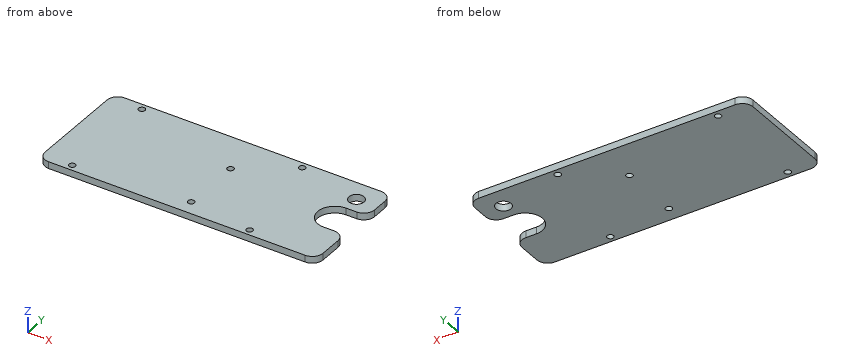
from build123d import *

# Parameters (mm, degrees)
F0_R     = 3.5
F1_DEPTH = 3.175
F3_R     = 5
F2_R     = 1.5
F4_DEPTH = 25


with BuildPart() as f1:
    # F0 (on Top) → F1 (new body)
    with BuildSketch(Plane.XY):
        with BuildLine():
            Line((65, 27), (-65, 27))
            Line((-65, 27), (-65, -27))
            Line((-65, -27), (65, -27))
            Line((65, -27), (65, -6.4))
            Line((65, -6.4), (55, -6.4))
            ThreePointArc((55, -6.4), (47, 1.6), (55, 9.6))
            Line((55, 9.6), (65, 9.6))
            Line((65, 9.6), (65, 27))
        make_face()
        with Locations((55, 17)):
            Circle(F0_R, mode=Mode.SUBTRACT)
    extrude(amount=F1_DEPTH)

    # F3
    f3_edges = [f1.edges().sort_by_distance(p)[0] for p in [
        (-65, -27, 1.5875),
        (-65, 27, 1.5875),
        (65, -27, 1.5875),
        (65, -6.4, 1.5875),
        (65, 9.6, 1.5875),
        (65, 27, 1.5875),
    ]]
    fillet(f3_edges, radius=F3_R)

    # F2 (on face) → F4 (cut)
    with BuildSketch(Plane.XY.offset(3.175)):
        with Locations((25, 24)):
            Circle(F2_R)
        with Locations((2, 8)):
            Circle(F2_R)
        with Locations((32, -24)):
            Circle(F2_R)
        with Locations((2, -20)):
            Circle(F2_R)
        with Locations((-50, 24)):
            Circle(F2_R)
        with Locations((-51, -24)):
            Circle(F2_R)
    extrude(amount=-F4_DEPTH, mode=Mode.SUBTRACT)


solid = f1.part
Could you check a few things on this model? Use its own coordinates, in mm. Round coordinates to 2 decimals unless told otherwise and drop trailing zeros. Loops run counter-clockwise (first coordinate to the right, second up) from the corner with the lowest first, then second, coordinate; pieces in that order, holes last. Notation, with made-up numbers: (-12, 33) -> (35, 33) arc R20 cw to (35, 47) -> close; hole circle Ø9 at (-24.75, 43). An arc over 180 degrees is marked (long way). Use CSV: the item, a comma, the result in double quotes.
(1) Suppose I cut it at B-B on x = 2. Write out the boundary of the cut face in (y, z) (3 decimals), plus the area to 3 significant figures.
Return value:
outline,"(-27, 0) -> (-21.5, 0) -> (-21.5, 3.175) -> (-27, 3.175) -> close; (-18.5, 0) -> (6.5, 0) -> (6.5, 3.175) -> (-18.5, 3.175) -> close; (9.5, 0) -> (27, 0) -> (27, 3.175) -> (9.5, 3.175) -> close"
area,"152 mm²"
(2) If I drill on probe 1 along Y at (x, z) = (55, 1.8); probe 2 along Y at (x, z) = (2, 2.25); probe 3 along Y at (x, z) = (59.5, 2.9), over which ranges is the centre line in solid material (lowest first)? Write a range as [from, to].
Return value:
probe 1,"y = [-27, -6.4], [9.6, 13.5], [20.5, 27]"
probe 2,"y = [-27, -21.5], [-18.5, 6.5], [9.5, 27]"
probe 3,"y = [-27, -6.4], [9.6, 27]"
(3) Suppose I cut it at D-D on x = 50. Write out the boundary of the cut face in (y, z) (3 decimals), plus the area to 3 significant figures.
Return value:
outline,"(-27, 0) -> (-4.645, 0) -> (-4.645, 3.175) -> (-27, 3.175) -> close; (7.845, 0) -> (27, 0) -> (27, 3.175) -> (7.845, 3.175) -> close"
area,"132 mm²"
(4) Will these pins go through, and if not, where does the flat tip stop? pin 1 Ø2.5 at (x, y) = (-50, 24) entering from -Z (3 decimals); pin 2 Ø4 at (x, y) = (32, -24) entering from +Z (3 decimals).
Return value:
pin 1,"passes through"
pin 2,"stops at z = 3.175"
(5) Suppose I cut it at C-C on z = 2.35. Write out the boundary of the cut face in (x, y).
Return value:
outline,"(-65, -22) arc R5 ccw to (-60, -27) -> (60, -27) arc R5 ccw to (65, -22) -> (65, -11.4) arc R5 ccw to (60, -6.4) -> (55, -6.4) arc R8 cw to (55, 9.6) -> (60, 9.6) arc R5 ccw to (65, 14.6) -> (65, 22) arc R5 ccw to (60, 27) -> (-60, 27) arc R5 ccw to (-65, 22) -> close; hole circle Ø3 at (-51, -24); hole circle Ø3 at (-50, 24); hole circle Ø3 at (2, -20); hole circle Ø3 at (2, 8); hole circle Ø3 at (25, 24); hole circle Ø3 at (32, -24); hole circle Ø7 at (55, 17)"
(6) Suppose I cut it at A-A on y = 17. Write out the boundary of the cut face in (x, z) (3 decimals).
Return value:
outline,"(-65, 0) -> (51.5, 0) -> (51.5, 3.175) -> (-65, 3.175) -> close; (58.5, 0) -> (65, 0) -> (65, 3.175) -> (58.5, 3.175) -> close"
